from build123d import *

# Parameters (mm, degrees)
TUBE001_R     = 9.5
TUBE001_R_2   = 8.25
TUBE001_DEPTH = 1
TUBE_R        = 12
TUBE_R_2      = 8.25
TUBE_DEPTH    = 2


with BuildPart() as tube001:
    # Tube001 → Tube001 (new body)
    with BuildSketch(Plane.XY):
        Circle(TUBE001_R)
        Circle(TUBE001_R_2, mode=Mode.SUBTRACT)
    extrude(amount=TUBE001_DEPTH)


with BuildPart() as fusion:
    # Tube → Tube (new body)
    with BuildSketch(Plane.XY.offset(1)):
        Circle(TUBE_R)
        Circle(TUBE_R_2, mode=Mode.SUBTRACT)
    extrude(amount=TUBE_DEPTH)

    # Fusion: union Tube001
    add(tube001.part)


solid = fusion.part
Input: part model. Units: mm. Frame: model coordinates. Give positions to 0.01 mm unless a question says otherwise; leave off trailing zeros. Order: outer loops, then holes, each group sorted by start corner. A loop starts at its lowest first (then second) coordinate and runs counter-clockwise, first axis right, second up.
Q1. Ray query, probe 1 along Y at (x, z) = (0, 2.2); probe 2 along Y at (x, z) = (7.5, 0.15); probe 3 along X at (y, z) = (5.5, 1.6). Return the intervals inside material, ascending.
Checked values:
probe 1: y = -12 to -8.25, 8.25 to 12
probe 2: y = -5.83 to -3.44, 3.44 to 5.83
probe 3: x = -10.67 to -6.15, 6.15 to 10.67
Q2. Draft query along X for faces 1 (the cylindrical face through (7.62, -3.16, 1.48)), 2 (the flat face through (9, 4, 1)), 3 (the cylindrical face through (4.38, -8.43, 0.49)). Return one class per face: +X half, -X half, draft (parallel to the pull), parting line (faces both ways), or undercut.
Checked values:
face 1: undercut
face 2: draft
face 3: parting line
Q3. Section D-D on z = 1.9. Output: boundary loops of the cut face in (x, y).
Checked values:
outline: circle Ø24 at (0, 0); hole circle Ø16.5 at (0, 0)
Q4. Section A-A on y = 0. Output: boundary loops of the cut face in (x, z), and give its area (3 significant figures).
Checked values:
outline: (-12, 1) - (-9.5, 1) - (-9.5, 0) - (-8.25, 0) - (-8.25, 3) - (-12, 3) - close; (8.25, 0) - (9.5, 0) - (9.5, 1) - (12, 1) - (12, 3) - (8.25, 3) - close
area: 17.5 mm2
Q5. Contact query for a flat-ended pin moving along its axis: pin 1 Ø1.5 at (y, z) = (7, 2) entering from +X. Output: stop coordinate, or through.
Checked values:
pin 1: stops at x = 10.24
Q6. Section C-C on z = 0.3. Output: boundary loops of the cut face in (x, y).
Checked values:
outline: circle Ø19 at (0, 0); hole circle Ø16.5 at (0, 0)
Q7. Section B-B on x = 4.25. Output: boundary loops of the cut face in (y, z), and give its area (3 significant figures).
Checked values:
outline: (-11.22, 1) - (-8.5, 1) - (-8.5, 0) - (-7.07, 0) - (-7.07, 3) - (-11.22, 3) - close; (7.07, 0) - (8.5, 0) - (8.5, 1) - (11.22, 1) - (11.22, 3) - (7.07, 3) - close
area: 19.5 mm2
